Input: part model. Units: mm. Frame: model coordinates. Face numbers are marked on the shaded views. A direction names the side the tool comes from. Give positions to 0.01 mm unless a question says otherwise; leave off trailing zeros. Order: outer loops, then holes, each group sorted by start corner. A loop starts at its lowest first (then second) coordinate and runs counter-clockwise, first axis right, second up. Notation, with made-up numbers: (5.25, -25) - (64.25, -25) arc R32 cw to (64.25, 9) - close; hole circle Ø9 at (40.5, -22.75). An arc over 180 degrees is marked (long way). Answer in a Markdown table with one row per item. Add a question column.
1. Access query for the marked faces 1 and 2. Directions: +Z, -Z, +X, -X, +Y, -Y. A direction counts if a zero-diameter tool reaches every point of the face in a straight line with its end or side. Return the directions, or none.
2. Section query D-D on z = 68. Return loops of the section in (x, y).
3. Section query A-A on x = 0. Return loops of the section in (y, z).
4. Contact query for flat-ended pins moving along their axis: pin 1 (6 mm diameter, centred on x = 9, y = 6.5, fed in from -Z); pin 2 (13.5 mm diameter, centred on x = 0, y = 0, fed in from -Z); pin 3 (4.5 mm diameter, centred on x = -12.84, z = 31.75, fed in from +Y). Output: stop coordinate, or through.
5. Ray query, line 1 (X direction, y = -18.5, z = 31.75); line 2 (Y direction, x = 11.5, z = 20); line 3 (X direction, y = -18, z = 82). Return the intervals inside material, ascending. Write a range as [from, to].
6. Section query B-B on z = 31.75. Return loops of the section in (x, y), and give its area (3 significant figures).
7. Section query C-C on x = -7.5. Return loops of the section in (y, z).
```python
from build123d import *

# Parameters (mm, degrees)
SKETCH1_R           = 11.254
BOSS_EXTRUDE1_DEPTH = 6.35
SKETCH2_W           = 35.208
SKETCH2_H           = 6.35
BOSS_EXTRUDE2_DEPTH = 102
SKETCH3_R           = 1.984375
CUT_EXTRUDE1_DEPTH  = 115.327080921


with BuildPart() as part:
    # Sketch1 → Boss-Extrude1 (new body)
    with BuildSketch(Plane.XY):
        with BuildLine():
            Line((-17.604, 0), (-17.604, -20.7))
            Line((-17.604, -20.7), (17.604, -20.7))
            Line((17.604, -20.7), (17.604, 0))
            ThreePointArc((17.604, 0), (0, 17.604), (-17.604, 0))
        make_face()
        Circle(SKETCH1_R, mode=Mode.SUBTRACT)
    extrude(amount=BOSS_EXTRUDE1_DEPTH)

    # Sketch2 → Boss-Extrude2 (add)
    with BuildSketch(Plane.XY.offset(6.35)):
        with Locations((0, -17.525)):
            Rectangle(SKETCH2_W, SKETCH2_H)
    extrude(amount=BOSS_EXTRUDE2_DEPTH)

    # Sketch3 → Cut-Extrude1 (cut, through all)
    with BuildSketch(Plane(origin=(0, -14.35, 0), x_dir=(1, 0, 0), z_dir=(0, 1, 0))):
        with Locations(Location((12.8415, -31.75, 0), (0, 0, 270))):
            Circle(SKETCH3_R)
        with Locations(Location((12.8415, -82.95, 0), (0, 0, 270))):
            Circle(SKETCH3_R)
        with Locations(Location((-12.8415, -82.95, 0), (0, 0, 90))):
            Circle(SKETCH3_R)
        with Locations(Location((-12.8415, -31.75, 0), (0, 0, 90))):
            Circle(SKETCH3_R)
    extrude(amount=-CUT_EXTRUDE1_DEPTH, mode=Mode.SUBTRACT)


solid = part.part
```
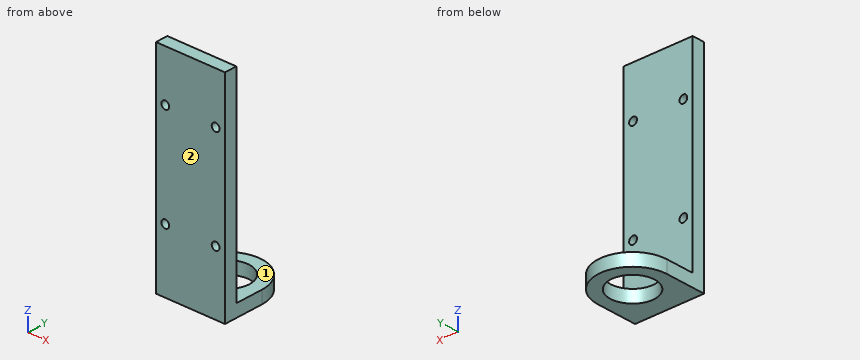
Answer:
| question | item | result |
|---|---|---|
| 1 | face 1 | +Z, +X, -X, +Y |
| 1 | face 2 | +Z, -Z, +X, -X, -Y |
| 2 | outline | (-17.6, -20.7) - (17.6, -20.7) - (17.6, -14.35) - (-17.6, -14.35) - close |
| 3 | outline | (-20.7, 0) - (-11.25, 0) - (-11.25, 6.35) - (-14.35, 6.35) - (-14.35, 108.35) - (-20.7, 108.35) - close; (11.25, 0) - (17.6, 0) - (17.6, 6.35) - (11.25, 6.35) - close |
| 4 | pin 1 | stops at z = 0 |
| 4 | pin 2 | passes through |
| 4 | pin 3 | stops at y = -14.35 |
| 5 | line 1 | x = [-17.6, -14.83], [-10.86, 10.86], [14.83, 17.6] |
| 5 | line 2 | y = [-20.7, -14.35] |
| 5 | line 3 | x = [-17.6, -14.58], [-11.1, 11.1], [14.58, 17.6] |
| 6 | outline | (-17.6, -20.7) - (-14.83, -20.7) - (-14.83, -14.35) - (-17.6, -14.35) - close; (-10.86, -20.7) - (10.86, -20.7) - (10.86, -14.35) - (-10.86, -14.35) - close; (14.83, -20.7) - (17.6, -20.7) - (17.6, -14.35) - (14.83, -14.35) - close |
| 6 | area | 173 mm² |
| 7 | outline | (-20.7, 0) - (-8.39, 0) - (-8.39, 6.35) - (-14.35, 6.35) - (-14.35, 108.35) - (-20.7, 108.35) - close; (8.39, 0) - (15.93, 0) - (15.93, 6.35) - (8.39, 6.35) - close |
